```python
from build123d import *

# Parameters (mm, degrees)
BOSS_EXTRUDE1_DEPTH = 0.889


with BuildPart() as part:
    # Sketch1 → Boss-Extrude1 (new body)
    with BuildSketch(Plane.XY):
        with BuildLine():
            Line((28.389672555, 3.075908507), (28.389672555, 13.075908507))
            ThreePointArc((28.389672555, 13.075908507), (28.267659086, 14.314732052), (27.906307587, 15.505948303))
            Line((27.906307587, 15.505948303), (22.833422555, 27.752976146))
            Line((22.833422555, 27.752976146), (21.245922555, 27.752976146))
            Line((21.245922555, 27.752976146), (16.173037524, 15.505948303))
            ThreePointArc((16.173037524, 15.505948303), (15.811686025, 14.314732052), (15.689672555, 13.075908507))
            Line((15.689672555, 13.075908507), (15.689672555, 3.075908507))
            ThreePointArc((15.689672555, 3.075908507), (22.039672555, -3.274091493), (28.389672555, 3.075908507))
        make_face()
    extrude(amount=BOSS_EXTRUDE1_DEPTH)

    # Sketch2 → Revolve1 (revolve)
    with BuildSketch(Plane.XY.offset(0.889), mode=Mode.PRIVATE) as revolve1_sk:
        with BuildLine():
            Line((22.039672555, 24.173793785), (22.039672555, 36.873793785))
            ThreePointArc((22.039672555, 36.873793785), (21.478406548, 36.641309793), (21.245922555, 36.080043785))
            Line((21.245922555, 36.080043785), (21.245922555, 24.967543785))
            ThreePointArc((21.245922555, 24.967543785), (21.478406548, 24.406277778), (22.039672555, 24.173793785))
        make_face()
    revolve(revolve1_sk.sketch.rotate(Axis((22.039672555, 24.173793785, 0.889), (0, 1, 0)), 270), axis=Axis((22.039672555, 24.173793785, 0.889), (0, 1, 0)))


solid = part.part
```
Geometry: final body of the model. Coordinates: model frame, mm. A direction names the side the tool comes from. Coordinates: 2 decimals unless noted, no trailing zeros. Order: outer loops, then holes, each group sorted by start corner. A loop starts at its lowest first (then second) coordinate and runs counter-clockwise, first axis right, second up. Notation, with made-up numbers: M 79,-12 L 114,-12 A33 ccw 114,16 Z; hole C -15,55.5 d2. An arc over 180 degrees is marked long. Answer in a Markdown table with one row per item. Add a question column.
Q1. Section query A-A on z = 0.6. Return the cut outline in (x, y), and give its area (3 significant figures).
Q2. Section query C-C on x = 24.25. Return the cut outline in (y, z), and give its area (3 significant figures).
Q3. Contact query for flat-ended pins moving along their axis: P1, Ø1, axis at x = 21, z = 1, coming from the +Y side; P2, Ø1, axis at y = 6.5, z = 1.5, coming from the +X side; P3, Ø6.5, axis at x = 21.5, y = 13, coming from the +Z side. Output: stop coordinate, or through.
Q4. Section query D-D on y = 31.5. Return the cut outline in (x, z).
Q5. Line query: L1, parallel to Z at x = 24.25, y = 15; L2, parallel to X at y = 26.5, z = 0.95; L3, parallel to Y at x = 19.5, z = 0.8. Output: solid intervals per line, ascending.
Q6. Reachability of faces 1 (the cylindrical face through (22, 30.45, 1.68)), 2 (the flat face through (18.745, 21.715, 0.438)) from +Z, -Z, +X, -X, +Y, -Y: full face, straight path, thin tool, end or side. Return the list, or none.
Q7. Section query B-B on y = 10.5. Return the cut outline in (x, z).
Completed:
| question | item | result |
|---|---|---|
| 1 | outline | M 15.69,3.08 A6.35 ccw 28.39,3.08 L 28.39,13.08 A6.35 ccw 27.91,15.51 L 22.83,27.75 L 22.78,27.75 L 22.78,36.08 A0.74 ccw 21.3,36.08 L 21.3,27.75 L 21.25,27.75 L 16.17,15.51 A6.35 ccw 15.69,13.08 Z |
| 1 | area | 315 mm2 |
| 2 | outline | M -2.88,0 L 24.33,0 L 24.33,0.89 L -2.88,0.89 Z |
| 2 | area | 24.2 mm2 |
| 3 | P1 | stops at y = 36.66 |
| 3 | P2 | passes through |
| 3 | P3 | stops at z = 0.89 |
| 4 | outline | C 22.04,0.89 d1.59 |
| 5 | L1 | z = 0 to 0.89 |
| 5 | L2 | x = 21.25 to 22.83 |
| 5 | L3 | y = -2.74 to 23.54 |
| 6 | face 1 | +Y |
| 6 | face 2 | +Z, -Z, -X, +Y |
| 7 | outline | M 15.69,0 L 28.39,0 L 28.39,0.89 L 15.69,0.89 Z |
